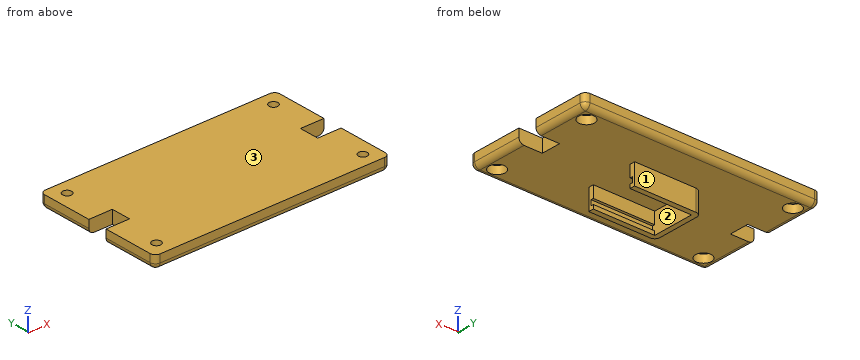
Autodesk Inventor part; units mm, degrees
ref_plane "YZ Plane" through (0, 0, 0) normal (1, 0, 0) x (0, 1, 0)
ref_plane "XZ Plane" through (0, 0, 0) normal (0, 1, 0) x (-1, 0, 0)
ref_plane "XY Plane" through (0, 0, 0) normal (0, 0, 1) x (1, 0, 0)
sketch "Náčrt1" plane through (0, 0, 0) normal (0, 0, 1) x (1, 0, 0)
  line L0 (0, 35) -> (0, -35)
  line L1 (-63, 0) -> (63, 0)
  line L2 (-45, 25) -> (45, 25)
  line L3 (45, 25) -> (45, -25)
  line L4 (45, -25) -> (-45, -25)
  line L5 (-45, -25) -> (-45, 25)
  point P0 (0, 0)
  dimension "d0" = 90
  dimension "d1" = 50
extrude "Vysunutí1" add sketch "Náčrt1" along normal blind 5
sketch "Náčrt4" plane through (0, 0, 0) normal (0, 0, -1) x (-1, 0, 0)
  line L0 (45, 25) -> (45, -25)
  line L1 (-45, 25) -> (45, 25)
  line L2 (-45, -25) -> (-45, 25)
  line L3 (45, -25) -> (-45, -25)
  line L4 (0, -35) -> (0, 35)
  line L5 (-63, 0) -> (63, 0)
  point P0 (0, 0)
  point P1 (-39.5, 19.5)
  dimension "d13" = 5.5
  dimension "d14" = 5.5
hole "Díra1" at (39.5, 19.5, 0) direction (0, 0, 1) diameter 3.4 end through all counterbore diameter 6.1 counterbore depth 3
mirror "Zrcadlit2" about plane through (0, 0, 0) normal (0, 1, 0) of "Díra1"
mirror "Zrcadlit3" about plane through (0, 0, 0) normal (1, 0, 0) of "Díra1", "Zrcadlit2"
fillet "Zaoblení2" radius 2 8 edges at (0, 25, 0) (45, 0, 0) (45, 25, 2.5) (0, -25, 0) (45, -25, 2.5) (-45, 0, 0) (-45, -25, 2.5) (-45, 25, 2.5)
sketch "Náčrt6" plane through (0, 0, 0) normal (0, 0, -1) x (-1, 0, 0)
  circle A0 centre (-39.5, 19.5) radius 3.05
  circle A1 centre (-39.5, -19.5) radius 3.05
  circle A2 centre (39.5, 19.5) radius 3.05
  circle A3 centre (39.5, -19.5) radius 3.05
  line L0 (43, -23) -> (-43, -23)
  line L1 (43, 23) -> (43, -23)
  line L2 (-43, 23) -> (43, 23)
  line L3 (-43, -23) -> (-43, 23)
  line L4 (-43, 23) -> (-45, 23)
  line L5 (-45, 23) -> (-45, -23)
  line L6 (-45, -23) -> (-43, -23)
  line L7 (-43, -23) -> (-43, 23)
  line L8 (-45, 3.75) -> (-36, 3.75)
  line L9 (-36, 3.75) -> (-36, -3.75)
  line L10 (-36, -3.75) -> (-45, -3.75)
  line L11 (-45, -3.75) -> (-45, 3.75)
  line L12 (-63, 0) -> (63, 0)
  point P0 (0, 0)
  dimension "d23" = 9
  dimension "d24" = 7.5
extrude "Vysunutí4" cut sketch "Náčrt6" against normal through all contours L10 L5 L12 L3 | L3 L12 L9 L10 | L12 L3 L8 L9 | L12 L5 L8 L3
mirror "Zrcadlit4" about plane through (0, 0, 0) normal (1, 0, 0) of "Vysunutí4"
sketch "Náčrt7" plane through (0, 0, 0) normal (0, 0, -1) x (-1, 0, 0)
  circle A0 centre (39.5, -19.5) radius 3.05
  circle A1 centre (39.5, 19.5) radius 3.05
  circle A2 centre (-39.5, -19.5) radius 3.05
  circle A3 centre (-39.5, 19.5) radius 3.05
  line L0 (43, -3.75) -> (36, -3.75)
  line L1 (36, -3.75) -> (36, 3.75)
  line L2 (36, 3.75) -> (43, 3.75)
  line L3 (43, 23) -> (43, 3.75)
  line L4 (-43, 23) -> (43, 23)
  line L5 (-43, 3.75) -> (-43, 23)
  line L6 (-43, 3.75) -> (-36, 3.75)
  line L7 (-36, 3.75) -> (-36, -3.75)
  line L8 (-36, -3.75) -> (-43, -3.75)
  line L9 (-43, -23) -> (-43, -3.75)
  line L10 (43, -23) -> (-43, -23)
  line L11 (43, -3.75) -> (43, -23)
  line L12 (43, 25) -> (-43, 25)
  line L13 (-43, -25) -> (43, -25)
  line L14 (-45, -3.75) -> (-45, -23)
  line L15 (45, -23) -> (45, -3.75)
  line L16 (45, 3.75) -> (45, 23)
  line L17 (-45, 23) -> (-45, 3.75)
  line L18 (0, -35) -> (0, 35)
  line L19 (-63, 0) -> (63, 0)
  line L20 (-12.75, 10) -> (12.75, 10)
  line L21 (12.75, 10) -> (12.75, -10)
  line L22 (12.75, -10) -> (-12.75, -10)
  line L23 (-12.75, -10) -> (-12.75, 10)
  line L24 (-10.75, 8) -> (10.75, 8)
  line L25 (10.75, 8) -> (10.75, -8)
  line L26 (10.75, -8) -> (-10.75, -8)
  line L27 (-10.75, -8) -> (-10.75, 8)
  line L28 (0, -8) -> (12.75, -8)
  line L29 (12.75, -8) -> (12.75, -10)
  line L30 (12.75, -10) -> (0, -10)
  line L31 (0, -10) -> (0, -8)
  line L32 (10.75, 0) -> (12.75, 0)
  line L33 (12.75, 0) -> (12.75, -10)
  line L34 (12.75, -10) -> (10.75, -10)
  line L35 (10.75, -10) -> (10.75, 0)
  point P0 (0, 0)
  dimension "d27" = 20
  dimension "d28" = 25.5
  dimension "d29" = 21.5
  dimension "d30" = 16
extrude "Vysunutí5" add sketch "Náčrt7" along normal blind 8 contours L21 L28 L25 L19 | L19 L25 L24 L18 L20 L21 | L22 L23 L19 L27 L26 L18 | L18 L26 L35 L22 | L21 L22 L35 L28 | L18 L24 L27 L19 L23 L20
sketch "Náčrt8" plane through (12.75, -10, 0) normal (1, 0, 0) x (0, 0, -1)
  line L0 (0, 2) -> (0, 18)
  line L1 (0, 2) -> (8, 2)
  line L2 (8, 18) -> (8, 2)
  line L3 (0, 18) -> (8, 18)
  line L4 (8, 18) -> (0, 18)
  line L5 (0, 18) -> (0, 2)
  line L6 (0, 2) -> (8, 2)
  line L7 (8, 2) -> (8, 18)
  point P0 (0, 10)
extrude "Vysunutí6" cut sketch "Náčrt8" against normal up to surface (2 mm away)
sketch "Náčrt9" plane through (12.75, 8, 0) normal (1, 0, 0) x (0, 0, -1)
  line L0 (8, -16) -> (0, -16)
  line L1 (0, -18) -> (0, -16)
  line L2 (0, -18) -> (8, -18)
  line L3 (8, -16) -> (8, -18)
  line L4 (0, 0) -> (8, 0)
  line L5 (8, 2) -> (8, 0)
  line L6 (0, 2) -> (8, 2)
  line L7 (0, 0) -> (0, 2)
  line L8 (4.5, 0) -> (6.5, 0)
  line L9 (6.5, 0) -> (6.5, 1)
  line L10 (6.5, 1) -> (4.5, 1)
  line L11 (4.5, 1) -> (4.5, 0)
  line L12 (-7.6, -8) -> (10.6, -8)
  point P0 (0, -8)
  dimension "d35" = 1
  dimension "d36" = 2
  dimension "d37" = 1.5
extrude "Vysunutí7" cut sketch "Náčrt9" against normal up to surface (23.5 mm away) contours L11 L10 L9 L4
mirror "Zrcadlit5" about plane through (0, 0, 0) normal (0, 1, 0) of "Vysunutí7"
fillet "Zaoblení3" radius 2 2 edges at (-12.75, 10, -4) (-12.75, -10, -4)
properties part number "tcs3200_gate_lid_3D tisk"
Work out the finished part from the listing and answer in its coordinate system (mm). Face numbers are marked on the shaded views. Give positions to 0.01 mm unless a question says otherwise; leave off trailing zeros. Loops run counter-clockwise (first coordinate to the right, second up) from the corner with the lowest first, then second, coordinate; pieces in that order, holes last. Notation, with made-up numbers: (-18.5, 12.25) -> (24.5, 12.25) arc R25 ccw to (24.5, 26.25) -> close; hole circle Ø11 at (9, -21.5). An arc over 180 degrees is marked (long way). Put each result on its own line as item: value. Start each with the question number.
Item 1: The part is cut by section A-A (y = -19.5). Give the vertices of the cut face in (x, z), then the cut area to 3 significant figures.
Item 2: The part is cut by section B-B (x = -39.5). Give the vertices of the cut face in (y, z).
Item 3: Find the intervals of material crossed by L1, parallel to X at y = 19.5, z = 3.8; L2, parallel to Y at x = 39.5, z = 4.25; L3, parallel to Y at x = 7, z = -2.75, in increasing order. Write a range as [from, to].
Item 4: The mould has two halves that part along Y. Classify the marked faces 1, 2 and 3: released by +Y, released by -Y, zero draft, split by the parting line, or undercut.
Item 5: The part is cut by section C-C (y = 2). Give the vertices of the cut face in (x, z).
Item 6: The part is cut by section D-D (z = -1.5). Give the vertices of the cut face in (x, y).
Item 7: Each of these flat-tipped pins is pushed along its axis until it touches: P1, Ø3, axis at x = -39.5, y = -19.5, coming from the +Z side (3 decimals); P2, Ø2, axis at x = -17, y = 18.5, coming from the -Z side; P3, Ø4.5, axis at x = -39.5, y = 19.5, coming from the -Z side; P4, Ø5, axis at x = -0.5, z = -5, coming from the -Y side. Where does it stop, or does it pass through?
Answers below:
1. outline: (-45, 2) arc R2 ccw to (-43, 0) -> (-42.55, 0) -> (-42.55, 3) -> (-41.2, 3) -> (-41.2, 5) -> (-45, 5) -> close; (-37.8, 3) -> (-36.45, 3) -> (-36.45, 0) -> (36.45, 0) -> (36.45, 3) -> (37.8, 3) -> (37.8, 5) -> (-37.8, 5) -> close; (41.2, 3) -> (42.55, 3) -> (42.55, 0) -> (43, 0) arc R2 ccw to (45, 2) -> (45, 5) -> (41.2, 5) -> close
1. area: 398 mm2
2. outline: (-25, 2) arc R2 ccw to (-23, 0) -> (-22.55, 0) -> (-22.55, 3) -> (-21.2, 3) -> (-21.2, 5) -> (-25, 5) -> close; (-17.8, 3) -> (-16.45, 3) -> (-16.45, 0) -> (-3.75, 0) -> (-3.75, 5) -> (-17.8, 5) -> close; (3.75, 0) -> (16.45, 0) -> (16.45, 3) -> (17.8, 3) -> (17.8, 5) -> (3.75, 5) -> close; (21.2, 3) -> (22.55, 3) -> (22.55, 0) -> (23, 0) arc R2 ccw to (25, 2) -> (25, 5) -> (21.2, 5) -> close
3. L1: [-45, -41.2], [-37.8, 37.8], [41.2, 45]
3. L2: [-25, -21.2], [-17.8, -3.75], [3.75, 17.8], [21.2, 25]
3. L3: [-10, -8], [8, 10]
4. face 1: released by +Y
4. face 2: undercut
4. face 3: zero draft
5. outline: (-36, 0) -> (-12.75, 0) -> (-12.75, -8) -> (-10.75, -8) -> (-10.75, 0) -> (36, 0) -> (36, 5) -> (-36, 5) -> close
6. outline: (-12.75, -8) arc R2 ccw to (-10.75, -10) -> (12.75, -10) -> (12.75, -8) -> (-10.75, -8) -> (-10.75, 8) -> (12.75, 8) -> (12.75, 10) -> (-10.75, 10) arc R2 ccw to (-12.75, 8) -> close
7. P1: through
7. P2: z = 0
7. P3: z = 3
7. P4: y = -10
